Autodesk Inventor part; units mm, degrees
ref_plane "YZ Plane" through (0, 0, 0) normal (1, 0, 0) x (0, 1, 0)
ref_plane "XZ Plane" through (0, 0, 0) normal (0, 1, 0) x (-1, 0, 0)
ref_plane "XY Plane" through (0, 0, 0) normal (0, 0, 1) x (1, 0, 0)
sketch "Sketch1" plane through (0, 0, 0) normal (0, 0, 1) x (1, 0, 0)
  line L0 (-40, 0) -> (-20, 0)
  line L1 (-20, 0) -> (-20, 5)
  line L2 (-20, 5) -> (-40, 5)
  line L3 (-40, 5) -> (-40, 0)
  arc A0 (20, 15) -> (-37, 5) centre (25.6963, -184.9189) ccw
  arc A1 (20, 9) -> (-25, 5) centre (32.8594, -390.7932) ccw
  line L4 (-37, 5) -> (-25, 5)
  line L5 (20, 15) -> (20, 9)
  line L6 (-20, 5) -> (-20, 5.6987)
  point P0 (0, 0)
  dimension "d0" = 20
  dimension "d9" = 5
  dimension "d11" = 40
  dimension "d13" = 20
  dimension "d14" = 5
  dimension "d16" = 10
  dimension "d17" = 3
  dimension "d19" = 6
  dimension "d20" = 40
  dimension "d21" = 200
  dimension "d22" = 400
  dimension "d24" = 12
extrude "Extrusion3" add sketch "Sketch1" along normal blind 5
sketch "Sketch3" plane through (-40, 0, 0) normal (0, -1, 0) x (1, 0, 0)
  line L0 (0, 5) -> (20, 5)
  line L1 (5, 5) -> (15, 5)
  line L2 (15, 5) -> (15, 0)
  line L3 (15, 0) -> (5, 0)
  line L4 (5, 0) -> (5, 5)
  line L5 (0, 0) -> (0, 5)
  point P0 (40, 0)
  dimension "d27" = 10
  dimension "d28" = 5
extrude "Extrusion4" cut sketch "Sketch3" against normal blind 3
chamfer "Chamfer1" distance 2 angle 45 1 edges at (-20, 5.6987, 2.5)
chamfer "Chamfer2" distance 3 angle 45 1 edges at (-40, 5, 2.5)
properties part number "CameraArm"
Here's how the part is built. I have some questions about the finished solid (model axes, mm). A direction names the side the tool comes from. Coordinates: 2 decimals unless noted, no trailing zeros. Order: outer loops, then holes, each group sorted by start corner. A loop starts at its lowest first (then second) coordinate and runs counter-clockwise, first axis right, second up.
1) Imagine slicing it at B-B on x = -23. List the corners of the cut face in (y, z) for me.
2) Imagine slicing it at C-C on y = 8. List the corners of the cut face in (x, z) for me.
3) I need wall thicknesses on line 1 (X direction, y = 1.25, z = 1.5); line 2 (Y direction, x = -8, z = 2.4); line 3 (Y direction, x = 11.5, z = 2.3). Which ranges of each line are inside material? Lowest first, please.
4) Which directions (+Z, -Z, +X, -X, +Y, -Y) give clear straight access to the entire face, cutting with the end or side of a thin tool? Please do faces 1 (the face through (-25, 1, 3)), 2 (the face through (-9.264, 12.002, 2.465)), 3 (the face through (-20, 2, 2)).
5) We'd pull the mould along X, two halves only. Please class faces 4 (the face through (-23, 0, 2)), 5 (the face through (-40, 1, 2)), 6 (the face through (-19.022, 4.813, 2.465)), 7 (the face through (-30, 3, 3)): +X half, -X half, draft (parallel to the pull), parting line (faces both ways), or undercut.
6) Will this pin go through, and if not, where does the flat tip stop? pin 1 (0.9 mm diameter, centred on y = 1, z = 3.5, fed in from +X).
Response values:
1. outline: (0, 0) - (9.06, 0) - (9.06, 5) - (0, 5) - close
2. outline: (-27.05, 0) - (1.81, 0) - (1.81, 5) - (-27.05, 5) - close
3. line 1: x = -40 to -35, -25 to -20
3. line 2: y = 7.11 to 12.22
3. line 3: y = 8.64 to 14.58
4. face 1: +Z, -Z, -Y
4. face 2: +Z, -Z, -X, +Y
4. face 3: +Z, -Z, +X, -Y
5. face 4: draft
5. face 5: -X half
5. face 6: +X half
5. face 7: undercut
6. pin 1: stops at x = -20
